from build123d import *

# Parameters (mm, degrees)
SKETCH1_R           = 38
SKETCH1_R_2         = 36
BOSS_EXTRUDE1_DEPTH = 16
SKETCH2_R           = 38
BOSS_EXTRUDE2_DEPTH = 2
CHAMFER1_SIZE       = 0.4
SKETCH3_R           = 5
BOSS_EXTRUDE3_DEPTH = 2
SKETCH4_R           = 3
BOSS_EXTRUDE4_DEPTH = 7
CHAMFER2_SIZE       = 0.4
CHAMFER3_SIZE       = 1


with BuildPart() as part:
    # Sketch1 → Boss-Extrude1 (new body)
    with BuildSketch(Plane(origin=(0, 0, 0), x_dir=(1, 0, 0), z_dir=(0, 1, 0))):
        Circle(SKETCH1_R)
        Circle(SKETCH1_R_2, mode=Mode.SUBTRACT)
    extrude(amount=BOSS_EXTRUDE1_DEPTH)

    # Sketch2 → Boss-Extrude2 (add)
    with BuildSketch(Plane(origin=(0, 16, 0), x_dir=(1, 0, 0), z_dir=(0, 1, 0))):
        Circle(SKETCH2_R)
    extrude(amount=BOSS_EXTRUDE2_DEPTH)

    # Chamfer1
    chamfer1_edges = [part.edges().sort_by_distance(p)[0] for p in [
        (-36, 16, 0),
        (-38, 0, 0),
        (-36, 0, 0),
    ]]
    chamfer(chamfer1_edges, length=CHAMFER1_SIZE)

    # Sketch3 → Boss-Extrude3 (add)
    with BuildSketch(Plane.XZ.offset(-16)):
        Circle(SKETCH3_R)
    extrude(amount=BOSS_EXTRUDE3_DEPTH)

    # Sketch4 → Boss-Extrude4 (add)
    with BuildSketch(Plane(origin=(0, 14, 0), x_dir=(-1, 0, 0), z_dir=(0, -1, 0))):
        Circle(SKETCH4_R)
    extrude(amount=BOSS_EXTRUDE4_DEPTH)

    # Chamfer2
    chamfer2_edges = [part.edges().sort_by_distance(p)[0] for p in [
        (-5, 16, 0),
        (-5, 14, 0),
        (3, 7, 0),
    ]]
    chamfer(chamfer2_edges, length=CHAMFER2_SIZE)

    # Chamfer3
    chamfer3_edges = [part.edges().sort_by_distance(p)[0] for p in [
        (-38, 18, 0),
    ]]
    chamfer(chamfer3_edges, length=CHAMFER3_SIZE)


solid = part.part
Can you work these out from the model? Positions are in its coordinate system, mm. A direction names the side the tool comes from. Coordinates: 2 decimals unless noted, no trailing zeros. Loops run counter-clockwise (first coordinate to the right, second up) from the corner with the lowest first, then second, coordinate; pieces in that order, holes last. Notation, with made-up numbers: M 21,-10.75 L 64,-10.75 A29 ccw 64,17.25 Z; hole C 62,89 d10. An arc over 180 degrees is marked long. Return JSON: item names as keys, results as strings. Group by question number.
Item 1: On a 3-axis mill with a long thin cutter (end or side, diameter ignored), from which of +Z, -Z, +X, -X, +Y, -Y can I reach the whole of each face in a straight line? I mean faces 1 (the flat face through (0, 16, 7)), 2 (the flat face through (-1, 18, -1)). Say none if no direction works.
Item 2: If I drill on L1, parallel to X at y = 12, z = 0; L2, parallel to X at y = 3.5, z = 0, over which ranges is the centre line in solid material (lowest first)? Write a range as from..to.
Item 3: Imagine slicing it at A-A (y = 9.5). Please give me the cut outline in (x, z), and give its area (3 significant figures).
Item 4: Imagine slicing it at D-D (y = 4.5). Please give me the cut outline in (x, z), and give its area (3 significant figures).
Item 5: Thinking about a two-plate mould opening in Z: for faces 3 (the flat face through (1, 14, -3)), 4 (the cylindrical face through (17.535, 8.584, 33.713)), 5 (the flat face through (-31, 0, -20)), which applies, released by +Z, released by -Z, zero draft, split by the parting line, or undercut?
Item 6: I'm going to push flat-ended pins straight in: pin 1 Ø8 at (x, y) = (-22.5, 2) entering from +Z; pin 2 Ø1.5 at (y, z) = (4.5, 16.5) entering from +X; pin 3 Ø4 at (x, z) = (-1, 0.5) entering from -Y. Where does each tip first touch, or does it pass through?
Verdict:
{
 "1": {"face 1": "-Y", "face 2": "+Z, -Z, +X, -X, +Y"},
 "2": {"L1": "x = -38..-36, -3..3, 36..38", "L2": "x = -38..-36, 36..38"},
 "3": {"outline": "C 0,0 d76; C 0,0 d6; hole C 0,0 d72", "area": "493 mm^2"},
 "4": {"outline": "C 0,0 d76; hole C 0,0 d72", "area": "465 mm^2"},
 "5": {"face 3": "undercut", "face 4": "split by the parting line", "face 5": "zero draft"},
 "6": {"pin 1": "stops at z = 33.19", "pin 2": "stops at x = 34.58", "pin 3": "stops at y = 7"}
}
